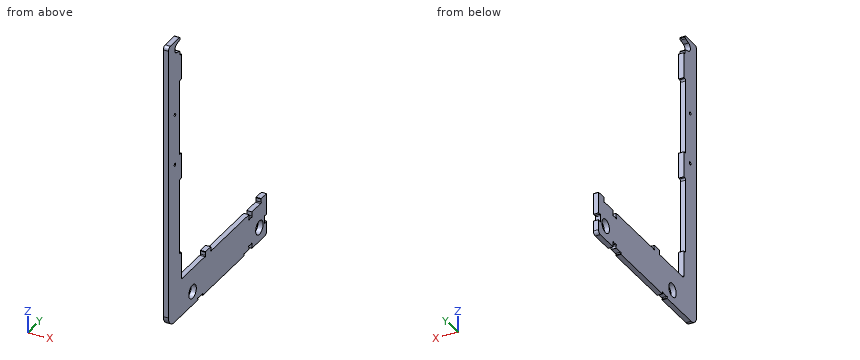
```python
from build123d import *

# Parameters (mm, degrees)
BOSS_EXTRUDE1_DEPTH = 15
FILLET1_R           = 30
SKETCH2_R           = 20.1
CUT_EXTRUDE1_DEPTH  = 820.456527218
FILLET2_R           = 6
SKETCH4_W           = 15
SKETCH4_H           = 30
BOSS_EXTRUDE2_DEPTH = 13
FILLET3_R           = 10
SKETCH5_W           = 20.5
SKETCH5_H           = 10.25
CUT_EXTRUDE3_DEPTH  = 820.456527218
SKETCH6_W           = 15.5
SKETCH6_H           = 16
CUT_EXTRUDE4_DEPTH  = 820.456527218
SKETCH7_W           = 5
SKETCH7_H           = 25.5
SKETCH7_H_2         = 26
CUT_EXTRUDE5_DEPTH  = 820.456527218
CHAMFER1_SIZE       = 1
SKETCH8_W           = 223.5
SKETCH8_H           = 10
CUT_EXTRUDE6_DEPTH  = 15
FILLET4_R           = 5
SKETCH9_R           = 2
CUT_EXTRUDE7_DEPTH  = 820.456527218
SKETCH10_R          = 2
CUT_EXTRUDE8_DEPTH  = 820.456527218
SKETCH11_R          = 2
CUT_EXTRUDE9_DEPTH  = 820.456527218
SKETCH12_R          = 2
CUT_EXTRUDE10_DEPTH = 820.456527218
BOSS_EXTRUDE3_DEPTH = 15
FILLET5_R           = 10
FILLET6_R           = 3
SKETCH14_R          = 4.25
CUT_EXTRUDE11_DEPTH = 866.513720284


with BuildPart() as part:
    # Sketch1 → Boss-Extrude1 (new body)
    with BuildSketch(Plane(origin=(0, 0, 0), x_dir=(0, 0, -1), z_dir=(1, 0, 0))):
        Polygon((-678, 0), (0, 0), (0, 460), (110, 460), (110, -69), (-678, -69), align=None)
    extrude(amount=BOSS_EXTRUDE1_DEPTH)

    # Fillet1
    fillet1_edges = [part.edges().sort_by_distance(p)[0] for p in [
        (7.5, -69, -110),
    ]]
    fillet(fillet1_edges, radius=FILLET1_R)

    # Sketch2 → Cut-Extrude1 (cut, through all)
    with BuildSketch(Plane(origin=(15, 0, 0), x_dir=(0, 0, -1), z_dir=(1, 0, 0))):
        with Locations((68.9, 421)):
            Circle(SKETCH2_R)
        with Locations((69.9, 61)):
            Circle(SKETCH2_R)
    extrude(amount=-CUT_EXTRUDE1_DEPTH, mode=Mode.SUBTRACT)

    # Fillet2
    fillet2_edges = [part.edges().sort_by_distance(p)[0] for p in [
        (7.5, 0, 0),
    ]]
    fillet(fillet2_edges, radius=FILLET2_R)

    # Sketch4 → Boss-Extrude2 (add)
    with BuildSketch(Plane.XY):
        with Locations((7.5, 445)):
            Rectangle(SKETCH4_W, SKETCH4_H)
        with Locations((7.5, 145)):
            Rectangle(SKETCH4_W, SKETCH4_H)
    extrude(amount=BOSS_EXTRUDE2_DEPTH)

    # Fillet3
    fillet3_edges = [part.edges().sort_by_distance(p)[0] for p in [
        (7.5, 460, -110),
    ]]
    fillet(fillet3_edges, radius=FILLET3_R)

    # Sketch5 → Cut-Extrude3 (cut, through all)
    with BuildSketch(Plane.ZY):
        with Locations((-60, 454.875)):
            Rectangle(SKETCH5_W, SKETCH5_H)
    extrude(amount=-CUT_EXTRUDE3_DEPTH, mode=Mode.SUBTRACT)

    # Sketch6 → Cut-Extrude4 (cut, through all)
    with BuildSketch(Plane(origin=(15, 0, 0), x_dir=(0, 0, -1), z_dir=(1, 0, 0))):
        with Locations((102.25, 372.5)):
            Rectangle(SKETCH6_W, SKETCH6_H)
        with Locations((7.75, 372.5)):
            Rectangle(SKETCH6_W, SKETCH6_H)
    extrude(amount=-CUT_EXTRUDE4_DEPTH, mode=Mode.SUBTRACT)

    # Sketch7 → Cut-Extrude5 (cut, through all)
    with BuildSketch(Plane.ZY):
        with Locations((-107.5, 351.75)):
            Rectangle(SKETCH7_W, SKETCH7_H)
        with Locations((-107.5, 102.5)):
            Rectangle(SKETCH7_W, SKETCH7_H_2)
    extrude(amount=-CUT_EXTRUDE5_DEPTH, mode=Mode.SUBTRACT)

    # Chamfer1
    chamfer1_edges = [part.edges().sort_by_distance(p)[0] for p in [
        (7.5, 430, 13),
        (7.5, 460, 13),
        (7.5, 130, 13),
        (7.5, 160, 13),
    ]]
    chamfer(chamfer1_edges, length=CHAMFER1_SIZE)

    # Sketch8 → Cut-Extrude6 (cut)
    with BuildSketch(Plane(origin=(15, 0, 0), x_dir=(0, 0, -1), z_dir=(1, 0, 0))):
        with Locations((-491.25, -5)):
            Rectangle(SKETCH8_W, SKETCH8_H)
        with Locations((-192.75, -5)):
            Rectangle(SKETCH8_W, SKETCH8_H)
    extrude(amount=-CUT_EXTRUDE6_DEPTH, mode=Mode.SUBTRACT)

    # Fillet4
    fillet4_edges = [part.edges().sort_by_distance(p)[0] for p in [
        (7.5, -10, 603),
        (7.5, -10, 379.5),
        (7.5, -10, 81),
        (7.5, -10, 304.5),
    ]]
    fillet(fillet4_edges, radius=FILLET4_R)

    # Sketch9 → Cut-Extrude7 (cut, through all)
    with BuildSketch(Plane(origin=(15, 0, 0), x_dir=(0, 0, -1), z_dir=(1, 0, 0))):
        with Locations((-0.707106781, 129.292893219)):
            Circle(SKETCH9_R)
        with Locations((-0.707106781, 160.707106781)):
            Circle(SKETCH9_R)
        with Locations((-0.707106781, 429.292893219)):
            Circle(SKETCH9_R)
    extrude(amount=-CUT_EXTRUDE7_DEPTH, mode=Mode.SUBTRACT)

    # Sketch10 → Cut-Extrude8 (cut, through all)
    with BuildSketch(Plane(origin=(15, 0, 0), x_dir=(0, 0, -1), z_dir=(1, 0, 0))):
        with Locations((50.457106781, 450.457106781)):
            Circle(SKETCH10_R)
        with Locations((69.542893219, 450.457106781)):
            Circle(SKETCH10_R)
    extrude(amount=-CUT_EXTRUDE8_DEPTH, mode=Mode.SUBTRACT)

    # Sketch11 → Cut-Extrude9 (cut, through all)
    with BuildSketch(Plane(origin=(15, 0, 0), x_dir=(0, 0, -1), z_dir=(1, 0, 0))):
        with Locations((14.792893219, 365.207106781)):
            Circle(SKETCH11_R)
        with Locations((14.792893219, 379.792893219)):
            Circle(SKETCH11_R)
        with Locations((95.207106781, 379.792893219)):
            Circle(SKETCH11_R)
        with Locations((95.207106781, 365.207106781)):
            Circle(SKETCH11_R)
    extrude(amount=-CUT_EXTRUDE9_DEPTH, mode=Mode.SUBTRACT)

    # Sketch12 → Cut-Extrude10 (cut, through all)
    with BuildSketch(Plane(origin=(15, 0, 0), x_dir=(0, 0, -1), z_dir=(1, 0, 0))):
        with Locations((105.707106781, 90.207106781)):
            Circle(SKETCH12_R)
        with Locations((105.707106781, 114.792893219)):
            Circle(SKETCH12_R)
        with Locations((105.707106781, 339.707106781)):
            Circle(SKETCH12_R)
    extrude(amount=-CUT_EXTRUDE10_DEPTH, mode=Mode.SUBTRACT)

    # Sketch13 → Boss-Extrude3 (add)
    with BuildSketch(Plane(origin=(15, 0, 0), x_dir=(0, 0, -1), z_dir=(1, 0, 0))):
        with BuildLine():
            Line((-678, -69), (-733, -69))
            Line((-733, -69), (-733, -7))
            Line((-733, -7), (-725.5, -7))
            Line((-725.5, -7), (-720.55324034, -25.378780397))
            ThreePointArc((-720.55324034, -25.378780397), (-708, -35), (-695.44675966, -25.378780397))
            Line((-695.44675966, -25.378780397), (-690.5, -7))
            Line((-690.5, -7), (-678, -7))
            Line((-678, -7), (-678, -69))
        make_face()
    extrude(amount=-BOSS_EXTRUDE3_DEPTH)

    # Fillet5
    fillet5_edges = [part.edges().sort_by_distance(p)[0] for p in [
        (7.5, -69, 733),
    ]]
    fillet(fillet5_edges, radius=FILLET5_R)

    # Fillet6
    fillet6_edges = [part.edges().sort_by_distance(p)[0] for p in [
        (7.5, -7, 733),
        (7.5, -7, 725.5),
        (7.5, -7, 690.5),
    ]]
    fillet(fillet6_edges, radius=FILLET6_R)

    # Sketch14 → Cut-Extrude11 (cut, through all)
    with BuildSketch(Plane(origin=(15, 0, 0), x_dir=(0, 0, -1), z_dir=(1, 0, 0))):
        with Locations((-513, -34)):
            Circle(SKETCH14_R)
        with Locations((-363, -34)):
            Circle(SKETCH14_R)
    extrude(amount=-CUT_EXTRUDE11_DEPTH, mode=Mode.SUBTRACT)


solid = part.part
```
Build history of the part. All positions in model axes, mm. Coordinates: 2 decimals unless noted, no trailing zeros. Order: outer loops, then holes, each group sorted by start corner. A loop starts at its lowest first (then second) coordinate and runs counter-clockwise, first axis right, second up. Notation, with made-up numbers: (-40, 4) -> (-29, 4) arc R17 cw to (-29, 36) -> close; hole circle Ø9 at (-9, 15). An arc over 180 degrees is marked (long way). Answer in a Markdown table with one row per item. Add a question column.
Q1. Band-saw the part on B-B, the plane z = 150.5. List the corners of the cut face in (x, y), then the cut area to 3 significant figures.
Q2. Drop flat-ended pins along their axis: pin 1 (6 mm diameter, centred on x = 2.5, z = 524, fed in from +Y); pin 2 (1 mm diameter, centred on x = 13.5, y = 346.5, fed in from +Z); pin 3 (7.5 mm diameter, centred on x = 10, z = 49, fed in from +Y). Give the stop position or say it passes through.
Q3. Band-saw the part on A-A, the plane y = 61. List the corners of the cut face in (x, z), then the cut area to 3 significant figures.
Q4. Wall check: line 1 along Y through (x, z) = (3.75, -69.9); line 2 along Y through (x, z) = (9.5, 363); line 3 along Z through (x, y) = (6.25, 420). Give the ranges that are in metal, low to high. Write a range as [from, to].
Q5. Band-saw the part on C-C, the plane x = 5.5. Give the number of separate pieces and of enclosed holes in the cut face, then the cut area to 3 significant figures.
Answers follow:
| question | item | result |
|---|---|---|
| 1 | outline | (0, -69) -> (15, -69) -> (15, -10) -> (0, -10) -> close |
| 1 | area | 885 mm^2 |
| 2 | pin 1 | y = -10 |
| 2 | pin 2 | z = 0 |
| 2 | pin 3 | y = 0 |
| 3 | outline | (0, -110) -> (15, -110) -> (15, -90) -> (0, -90) -> close; (0, -49.8) -> (15, -49.8) -> (15, 0) -> (0, 0) -> close |
| 3 | area | 1,050 mm^2 |
| 4 | line 1 | [-69, 40.9], [81.1, 400.92], [441.08, 448.49] |
| 4 | line 2 | [-69, -38.25], [-29.75, 0] |
| 4 | line 3 | [-110, -88.98], [-48.82, 0] |
| 5 | separate pieces | 1 |
| 5 | enclosed holes | 4 |
| 5 | area | 100,000 mm^2 |
